from build123d import *

# Parameters (mm, degrees)
SKETCH1_W           = 2
SKETCH1_H           = 76
BOSS_EXTRUDE1_DEPTH = 15
SKETCH2_W           = 10
SKETCH2_H           = 3
BOSS_EXTRUDE2_DEPTH = 12
SKETCH3_R           = 2.6
CUT_EXTRUDE1_DEPTH  = 12
FILLET1_R           = 5
SCALE1_SCALE        = 0.7


with BuildPart() as part:
    # Sketch1 → Boss-Extrude1 (new body)
    with BuildSketch(Plane(origin=(0, 0, 0), x_dir=(0, 1, 0), z_dir=(0, 0, 1))):
        Rectangle(SKETCH1_W, SKETCH1_H)
    extrude(amount=-BOSS_EXTRUDE1_DEPTH)

    # Sketch2 → Boss-Extrude2 (add)
    with BuildSketch(Plane.XZ.offset(1)):
        with Locations((0, -3.8)):
            Rectangle(SKETCH2_W, SKETCH2_H)
        with Locations((0, -11.3)):
            Rectangle(SKETCH2_W, SKETCH2_H)
    extrude(amount=BOSS_EXTRUDE2_DEPTH)

    # Sketch3 → Cut-Extrude1 (cut)
    with BuildSketch(Plane.XY.offset(-2.3)):
        with Locations((0, -7)):
            Circle(SKETCH3_R)
    extrude(amount=-CUT_EXTRUDE1_DEPTH, mode=Mode.SUBTRACT)

    # Fillet1
    fillet1_edges = [part.edges().sort_by_distance(p)[0] for p in [
        (-5, -13, -11.3),
        (5, -13, -11.3),
        (5, -13, -3.8),
        (-5, -13, -3.8),
    ]]
    fillet(fillet1_edges, radius=FILLET1_R - 0.0001)  # a hair under: the kernel refuses the full size


with BuildPart() as part_1:
    # Scale1: scaled about (0, -1.204695158, -7.509404587)
    add(part.part.scale(SCALE1_SCALE).moved(Location((0, -0.361408547, -2.252821376))))


solid = part_1.part
The model under review builds one solid part; all positions refer to its coordinate system, in mm. A direction names the side the tool comes from. Give positions to 0.01 mm unless a question says otherwise; leave off trailing zeros. Order: outer loops, then holes, each group sorted by start corner. A loop starts at its lowest first (then second) coordinate and runs counter-clockwise, first axis right, second up. Notation, with made-up numbers: M 64.25,0.25 L 88.25,0.25 A9 ccw 88.25,11.25 Z; hole C 16,-2 d2. An arc over 180 degrees is marked long. Answer in a Markdown table with one row per item. Add a question column.
1. For pin 1 Ø5 at (y, z) = (-6.5, -6) entering from +X; pin 2 Ø2 at (x, y) = (0, -7.5) entering from -Z; pin 3 Ø0.6 at (y, z) = (-4, -10.5) entering from -X, all flat-tipped, find the tip position at first contact; note any pin that passes through.
2. Mouldability with a two-part tool opening along X and no side actions: class faces 4 (the flat face through (-3.5, -3, -5)), 5 (the flat face through (0, 0.339, -7)), 6 (the cylindrical face through (0.98, -3.73, -4.9)), 7 (the cylindrical face through (0.98, -3.73, -10.15)) as released by +X, released by -X, zero draft, split by the parting line, or undercut.
3. To check wall thickness, follow line 1 along Y through (x, z) = (0, -10.2); line 2 along Y through (x, z) = (7, -3); line 3 along Z through (x, y) = (2.5, -1.25). State the ranges of each line that lie inside material, in increasing order.
4. Machinability: for faces 1 (the flat face through (0, -3, -9.113)), 2 (the flat face through (0, -3, -11.213)), 3 (the flat face through (0, -3, -3.863)), which of the approach directions +Z, -Z, +X, -X, +Y, -Y give a long, thin tool a straight path to every point of the face, cutting with its end or side? Answer none if there is none.
5. Add section A-A on x = 18.5. State the section outline as (y, z) points, plus the area to 3 significant figures.
The answers:
| question | item | result |
|---|---|---|
| 1 | pin 1 | x = 3.5 |
| 1 | pin 2 | z = -11.21 |
| 1 | pin 3 | x = -3.5 |
| 2 | face 4 | released by -X |
| 2 | face 5 | zero draft |
| 2 | face 6 | undercut |
| 2 | face 7 | undercut |
| 3 | line 1 | -9.46 to -7.08, -3.44 to 0.34 |
| 3 | line 2 | -1.06 to 0.34 |
| 3 | line 3 | -11.21 to -9.11, -5.96 to -3.86 |
| 4 | face 1 | +X, -X, -Y |
| 4 | face 2 | -Z, +X, -X, -Y |
| 4 | face 3 | +Z, +X, -X, -Y |
| 5 | outline | M -1.06,-12.75 L 0.34,-12.75 L 0.34,-2.25 L -1.06,-2.25 Z |
| 5 | area | 14.7 mm2 |
